Source: CAD feature listing. Evaluate the final solid. Frame: model axes, mm. Face numbers are marked on the shaded views. A direction names the side the tool comes from. Coordinates: 2 decimals unless noted, no trailing zeros. Loops run counter-clockwise (first coordinate to the right, second up) from the corner with the lowest first, then second, coordinate; pieces in that order, holes last. Notation, with made-up numbers: (10.25, -3.5) - (55.25, -3.5) arc R28 cw to (55.25, 20.5) - close; hole circle Ø4 at (40.25, 13). An arc over 180 degrees is marked (long way). Use CSV: the item, a comma, the result in double quotes. Start each with the question number.
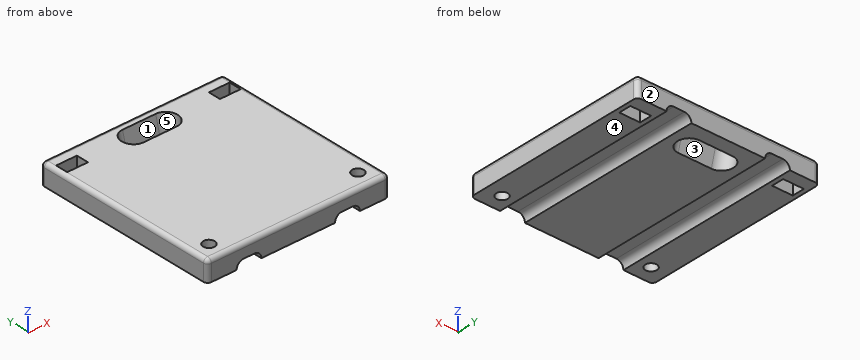
```python
from build123d import *

# Parameters (mm, degrees)
SKETCH1_W                       = 44
SKETCH1_H                       = 45
BASE_DEPTH                      = 5
WIRE_GROOVES_DEPTH              = 51.338851795
SCREW_INSERTION_HOLE_DEPTH      = 33.181634738
SCREW_INSERTION_HOLE_DEPTH_BACK = 33.181634738
SKETCH5_W                       = 5
SKETCH5_H                       = 3
ZIP_TIE_SLOTS_DEPTH             = 32.862987933
SKETCH6_R                       = 1.4
MOUNT_CLAMPING_HOLES_DEPTH      = 32.862987933
EDGE_FILLETS_R                  = 1


with BuildPart() as part:
    # Sketch1 → Base (new body)
    with BuildSketch(Plane.XY):
        Rectangle(SKETCH1_W, SKETCH1_H)
    extrude(amount=BASE_DEPTH)

    # Sketch2 → Wire Grooves (cut, through all)
    with BuildSketch(Plane(origin=(0, 22.5, 0), x_dir=(1, 0, 0), z_dir=(0, 1, 0))):
        with BuildLine():
            Line((-14.9, 0), (-8.9, 0))
            ThreePointArc((-8.9, 0), (-9.397918472, -1.202081528), (-10.6, -1.7))
            Line((-10.6, -1.7), (-13.2, -1.7))
            ThreePointArc((-13.2, -1.7), (-14.402081528, -1.202081528), (-14.9, 0))
        make_face()
        with BuildLine():
            Line((13.2, -1.7), (10.6, -1.7))
            ThreePointArc((10.6, -1.7), (9.397918472, -1.202081528), (8.9, 0))
            Line((8.9, 0), (14.9, 0))
            ThreePointArc((14.9, 0), (14.402081528, -1.202081528), (13.2, -1.7))
        make_face()
    extrude(amount=-WIRE_GROOVES_DEPTH, mode=Mode.SUBTRACT)

    # Sketch3 → Screw Insertion Hole (cut, two sides: drawn at the far end of the back side and taken through both)
    with BuildSketch(Plane(origin=(0, 0.596130014, 4.269237963), x_dir=(-1, 0, 0), z_dir=(0, -0.25881904510252135, -0.9659258262890681)).offset(-SCREW_INSERTION_HOLE_DEPTH_BACK)):
        with BuildLine():
            Line((-4, 19.042473808), (4, 19.042473808))
            ThreePointArc((4, 19.042473808), (6.75, 16.292473808), (4, 13.542473808))
            Line((4, 13.542473808), (-4, 13.542473808))
            ThreePointArc((-4, 13.542473808), (-6.75, 16.292473808), (-4, 19.042473808))
        make_face()
    extrude(amount=SCREW_INSERTION_HOLE_DEPTH + SCREW_INSERTION_HOLE_DEPTH_BACK, mode=Mode.SUBTRACT)

    # Sketch5 → Zip Tie Slots (cut, through all)
    with BuildSketch(Plane(origin=(0, 0, 0), x_dir=(-1, 0, 0), z_dir=(0, 0, -1))):
        with Locations((-18.45, 18)):
            Rectangle(SKETCH5_W, SKETCH5_H)
        with Locations((18.45, 18)):
            Rectangle(SKETCH5_W, SKETCH5_H)
    extrude(amount=-ZIP_TIE_SLOTS_DEPTH, mode=Mode.SUBTRACT)

    # Sketch6 → Mount Clamping Holes (cut, through all)
    with BuildSketch(Plane(origin=(0, 0, 0), x_dir=(-1, 0, 0), z_dir=(0, 0, -1))):
        with Locations((-18, -18.5)):
            Circle(SKETCH6_R)
        with Locations(Location((18, -18.5, 0), (0, 0, 180))):
            Circle(SKETCH6_R)
    extrude(amount=-MOUNT_CLAMPING_HOLES_DEPTH, mode=Mode.SUBTRACT)

    # Edge Fillets
    edge_fillets_edges = [part.edges().sort_by_distance(p)[0] for p in [
        (-22, 0, 5),
        (0, -22.5, 5),
        (22, 0, 5),
        (22, -22.5, 2.5),
        (-22, -22.5, 2.5),
        (-22, 22.5, 2.5),
        (22, 22.5, 2.5),
        (0, 22.5, 5),
    ]]
    fillet(edge_fillets_edges, radius=EDGE_FILLETS_R)


solid = part.part
```
(1) Pin query (flat end, axial travel): pin 1 Ø3 at (x, y) = (12.5, 5.5) entering from -Z; pin 2 Ø0.8 at (x, y) = (-12, -6.5) entering from -Z. Return the tip coordinate at first contact, or that it passes through.
(2) Section A-A on y = -18.5. Output: boundary loops of the cut face in (x, z).
(3) Ray query, line 1 (Y direction, x = -18, z = 1.35); line 2 (X direction, y = 17, z = 0.8); line 3 (Y direction, x = -17, z = 1.4). Return the intervals inside material, ascending. Write a range as [from, to].
(4) Section C-C on x = 18. Output: boundary loops of the cut face in (y, z).
(5) Reachability of the marked faces 3, 4 and 5 from +Z, -Z, +X, -X, +Y, -Y: full face, straight path, thin tool, end or side. Return the list, or none.
(6) Section B-B on x = -3. Output: boundary loops of the cut face in (y, z), plus the area to 3 significant figures.
(7) Draft query along X for the marked faces 1 and 2. Return one class per face: released by +X, released by -X, zero draft, split by the parting line, or undercut.
(8) Section D-D on z = 1.1. State how many separate pieces and enclosed holes the cut face has, plus the area to 3 significant figures.
Solution:
1,pin 1,"stops at z = 1.5"
1,pin 2,"stops at z = 1.7"
2,outline,"(-22, 0) - (-19.4, 0) - (-19.4, 5) - (-21, 5) arc R1 ccw to (-22, 4) - close; (-16.6, 0) - (-14.9, 0) arc R1.7 cw to (-13.2, 1.7) - (-10.6, 1.7) arc R1.7 cw to (-8.9, 0) - (8.9, 0) arc R1.7 cw to (10.6, 1.7) - (13.2, 1.7) arc R1.7 cw to (14.9, 0) - (16.6, 0) - (16.6, 5) - (-16.6, 5) - close; (19.4, 0) - (22, 0) - (22, 4) arc R1 ccw to (21, 5) - (19.4, 5) - close"
3,line 1,"y = [-22.5, -19.9], [-17.1, 16.5], [19.5, 22.5]"
3,line 2,"x = [-22, -20.95], [-15.95, -14.7], [-9.1, -6.71], [6.71, 9.1], [14.7, 15.95], [20.95, 22]"
3,line 3,"y = [-22.5, -19.48], [-17.52, 16.5], [19.5, 22.5]"
4,outline,"(-22.5, 0) - (-19.9, 0) - (-19.9, 5) - (-21.5, 5) arc R1 ccw to (-22.5, 4) - close; (-17.1, 0) - (16.5, 0) - (16.5, 5) - (-17.1, 5) - close; (19.5, 0) - (22.5, 0) - (22.5, 4) arc R1 ccw to (21.5, 5) - (19.5, 5) - close"
5,face 3,"-Z"
5,face 4,"-Z, +X, -X, +Y, -Y"
5,face 5,"none"
6,outline,"(-22.5, 0) - (13.47, 0) - (14.81, 5) - (-21.5, 5) arc R1 ccw to (-22.5, 4) - close; (19.17, 0) - (22.5, 0) - (22.5, 4) arc R1 ccw to (21.5, 5) - (20.51, 5) - close"
6,area,"196 mm²"
7,face 1,"undercut"
7,face 2,"zero draft"
8,separate pieces,"3"
8,enclosed holes,"5"
8,area,"1,400 mm²"
